Input: part model. Units: mm. Frame: model coordinates. A direction names the side the tool comes from. Give positions to 0.01 mm unless a question says otherwise; leave off trailing zeros. Write each loop counter-clockwise with the first axis right and the second up, starting at its lowest first coordinate (ties: lowest second). Pieces come first, ordered by that corner, then holes.
```python
from build123d import *

# Parameters (mm, degrees)
BOSS_EXTRUDE1_DEPTH = 2
CHAMFER1_SIZE       = 0.05
BOSS_EXTRUDE2_DEPTH = 0.5
CUT_EXTRUDE1_DEPTH  = 15.484682492
SKETCH5_R           = 1
CUT_EXTRUDE2_DEPTH  = 9.539796483


with BuildPart() as part:
    # Sketch1 → Boss-Extrude1 (new, symmetric)
    with BuildSketch(Plane.XY):
        with BuildLine():
            Line((0, 0), (2.405, 0))
            ThreePointArc((2.405, 0), (2.443345275, 0.133049905), (2.546618218, 0.225285129))
            Line((2.546618218, 0.225285129), (4.891908909, 1.353574355))
            ThreePointArc((4.891908909, 1.353574355), (5.408273626, 1.814750474), (5.6, 2.48))
            Line((5.6, 2.48), (5.6, 7.38))
            Line((5.6, 7.38), (5, 7.38))
            Line((5, 7.38), (5, 2.48))
            Line((5, 2.48), (0, 2.48))
            Line((0, 2.48), (0, 0))
        make_face()
    boss_extrude1 = extrude(amount=BOSS_EXTRUDE1_DEPTH, both=True)

    # Mirror1: Boss-Extrude1 across plane
    add(boss_extrude1.mirror(Plane(origin=(0, 0, 0), x_dir=(0, 0, 1), z_dir=(1, 0, 0))))

    # Chamfer1
    chamfer1_edges = [part.edges().sort_by_distance(p)[0] for p in [
        (5, 2.48, 0),
        (-5, 2.48, 0),
    ]]
    chamfer(chamfer1_edges, length=CHAMFER1_SIZE)

    # Sketch3 → Boss-Extrude2 (add, symmetric)
    with BuildSketch(Plane.XY):
        with BuildLine():
            Line((2.546618218, 0.225285129), (4.233522805, 0))
            ThreePointArc((4.233522805, 0), (6.206510258, 0.776923649), (6.585860055, 2.863160351))
            Line((6.585860055, 2.863160351), (5.6, 5.76))
            Line((5.6, 5.76), (5.6, 2.48))
            ThreePointArc((5.6, 2.48), (5.408273626, 1.814750474), (4.891908909, 1.353574355))
            Line((4.891908909, 1.353574355), (2.546618218, 0.225285129))
        make_face()
    boss_extrude2 = extrude(amount=BOSS_EXTRUDE2_DEPTH, both=True)

    # Mirror2: Boss-Extrude2 across plane
    add(boss_extrude2.mirror(Plane(origin=(0, 0, 0), x_dir=(0, 0, 1), z_dir=(1, 0, 0))))

    # Sketch4 → Cut-Extrude1 (cut, through all)
    with BuildSketch(Plane(origin=(5.6, 0, 0), x_dir=(0, 0, -1), z_dir=(1, 0, 0))):
        with BuildLine():
            Line((0.375, 6.42), (0.375, 7.38))
            Line((0.375, 7.38), (-0.375, 7.38))
            Line((-0.375, 7.38), (-0.375, 6.42))
            ThreePointArc((-0.375, 6.42), (0, 6.045), (0.375, 6.42))
        make_face()
    extrude(amount=-CUT_EXTRUDE1_DEPTH, mode=Mode.SUBTRACT)

    # Sketch5 → Cut-Extrude2 (cut, through all)
    with BuildSketch(Plane(origin=(0, 2.48, 0), x_dir=(1, 0, 0), z_dir=(0, 1, 0))):
        with Locations(Location((0, 0, 0), (0, 0, 180))):
            Circle(SKETCH5_R)
    extrude(amount=-CUT_EXTRUDE2_DEPTH, mode=Mode.SUBTRACT)


solid = part.part
```
Item 1: Section D-D (z = 1.6). Return loops of the section in (x, y) (3 decimals), and give its area (3 significant figures).
Item 2: Section B-B (z = 0). Return loops of the section in (x, y) (3 decimals), and give its area (3 significant figures).
Item 3: Pin query (flat end, axial travel): pin 1 (2 mm diameter, centred on y = 4, z = 0.5, fed in from -X); pin 2 (1.2 mm diameter, centred on y = 5.5, z = -1, fed in from +X); pin 3 (1.5 mm diameter, centred on x = -4, y = 4.5, fed in from +Z); pin 4 (2 mm diameter, centred on y = 6, z = 0, fed in from -X). Return the tip coordinate at first contact, or that it passes through.
Item 4: Set-up query: faces 1 (the cylindrical face through (5.4, 1.8, 1.3)), 2 (the cylindrical face through (5.4, 1.8, -1.2)), 3 (the flat face through (-5, 5, 0)), 4 (the flat face through (-6, 2, -0.5)). Return all of +Z, -Z, +X, -X, +Y, -Y with unobstructed straight access to the full face (end or side cutting, diameter ignored); none if empty.
Item 5: Section A-A (x = 0). Return loops of the section in (y, z).
Item 6: Section C-C (y = 3). Return loops of the section in (x, z).
Item 7: Ray query, line 1 (Z direction, x = 0, y = 1.9); line 2 (X direction, y = 2.75, z = 1.6); line 3 (Y direction, x = 2, z = 0.9). Return the intervals inside material, ascending.
Item 8: Mould query, pull axis Z, two halves, no side actions, for faces 5 (the cylindrical face through (-5.4, 1.8, 1.3)), 6 (the flat face through (6, 2, 0.5)), 7 (the flat face through (6, 2, -0.5)), 8 (the cylindrical face through (0, 1, -1)). Classes: +Z half, -Z half, draft (parallel to the pull), parting line (faces both ways), or undercut.
Solved:
1. outline: (-5.6, 2.48) arc R1.25 ccw to (-4.892, 1.354) - (-2.547, 0.225) arc R0.25 cw to (-2.405, 0) - (2.405, 0) arc R0.25 cw to (2.547, 0.225) - (4.892, 1.354) arc R1.25 ccw to (5.6, 2.48) - (5.6, 7.38) - (5, 7.38) - (5, 2.53) - (4.95, 2.48) - (-4.95, 2.48) - (-5, 2.53) - (-5, 7.38) - (-5.6, 7.38) - close
1. area: 27.5 mm2
2. outline: (-6.586, 2.863) arc R2.18 ccw to (-4.234, 0) - (-2.547, 0.225) arc R0.25 cw to (-2.405, 0) - (-1, 0) - (-1, 2.48) - (-4.95, 2.48) - (-5, 2.53) - (-5, 6.045) - (-5.6, 6.045) - (-5.6, 5.76) - close; (1, 0) - (2.405, 0) arc R0.25 cw to (2.547, 0.225) - (4.234, 0) arc R2.18 ccw to (6.586, 2.863) - (5.6, 5.76) - (5.6, 6.045) - (5, 6.045) - (5, 2.53) - (4.95, 2.48) - (1, 2.48) - close
2. area: 33.8 mm2
3. pin 1: stops at x = -6.54
3. pin 2: stops at x = 5.8
3. pin 3: passes through
3. pin 4: stops at x = -5.86
4. face 1: +Z, +X, -Y
4. face 2: -Z, +X, -Y
4. face 3: +Z, -Z, +Y
4. face 4: -Z, -X, -Y
5. outline: (0, -2) - (2.48, -2) - (2.48, -1) - (0, -1) - close; (0, 1) - (2.48, 1) - (2.48, 2) - (0, 2) - close
6. outline: (-6.54, -0.5) - (-5.6, -0.5) - (-5.6, -2) - (-5, -2) - (-5, 2) - (-5.6, 2) - (-5.6, 0.5) - (-6.54, 0.5) - close; (5, -2) - (5.6, -2) - (5.6, -0.5) - (6.54, -0.5) - (6.54, 0.5) - (5.6, 0.5) - (5.6, 2) - (5, 2) - close
7. line 1: z = -2 to -1, 1 to 2
7. line 2: x = -5.6 to -5, 5 to 5.6
7. line 3: y = 0 to 2.48
8. face 5: draft
8. face 6: +Z half
8. face 7: -Z half
8. face 8: undercut
